```python
from build123d import *

# Parameters (mm, degrees)
CYLINDER1528_R     = 1.5
CYLINDER1528_DEPTH = 100
CYLINDER1527_R     = 1.5
CYLINDER1527_DEPTH = 100
CYLINDER1526_R     = 1.5
CYLINDER1526_DEPTH = 32
CYLINDER1525_R     = 1.5
CYLINDER1525_DEPTH = 32
BOX520_W           = 200
BOX520_H           = 100
BOX520_DEPTH       = 100
BOX519_W           = 200
BOX519_H           = 100
BOX519_DEPTH       = 100
CYLINDER1518_R     = 4
CYLINDER1518_DEPTH = 100
CYLINDER1519_R     = 4
CYLINDER1519_DEPTH = 100
CYLINDER1520_R     = 4
CYLINDER1520_DEPTH = 100
CYLINDER1521_R     = 4
CYLINDER1521_DEPTH = 100
CYLINDER1522_R     = 4
CYLINDER1522_DEPTH = 100
CYLINDER1523_R     = 4
CYLINDER1523_DEPTH = 100
CYLINDER1524_R     = 4
CYLINDER1524_DEPTH = 100
CYLINDER1517_R     = 4
CYLINDER1517_DEPTH = 100
CYLINDER1510_R     = 1.5
CYLINDER1510_DEPTH = 100
CYLINDER1511_R     = 1.5
CYLINDER1511_DEPTH = 100
CYLINDER1512_R     = 1.5
CYLINDER1512_DEPTH = 100
CYLINDER1513_R     = 1.5
CYLINDER1513_DEPTH = 100
CYLINDER1514_R     = 1.5
CYLINDER1514_DEPTH = 100
CYLINDER1515_R     = 1.5
CYLINDER1515_DEPTH = 100
CYLINDER1516_R     = 1.5
CYLINDER1516_DEPTH = 100
CYLINDER1509_R     = 1.5
CYLINDER1509_DEPTH = 100
CYLINDER1508_R     = 59
CYLINDER1508_DEPTH = 4


with BuildPart() as obj1:
    # Cylinder1528 → Cylinder1528 (new body)
    with BuildSketch(Plane(origin=(14, 0, -60), x_dir=(1, 0, 0), z_dir=(0, 0, 1))):
        Circle(CYLINDER1528_R)
    extrude(amount=CYLINDER1528_DEPTH)


with BuildPart() as obj2:
    # Cylinder1527 → Cylinder1527 (new body)
    with BuildSketch(Plane(origin=(90, 0, -60), x_dir=(1, 0, 0), z_dir=(0, 0, 1))):
        Circle(CYLINDER1527_R)
    extrude(amount=CYLINDER1527_DEPTH)

    # Compound900: union obj1
    add(obj1.part)


with BuildPart() as obj3:
    # Cylinder1526 → Cylinder1526 (new body)
    with BuildSketch(Plane(origin=(78, 41, -42), x_dir=(1, 0, 0), z_dir=(0, 0, 1))):
        Circle(CYLINDER1526_R)
    extrude(amount=CYLINDER1526_DEPTH)


with BuildPart() as compound899:
    # Cylinder1525 → Cylinder1525 (new body)
    with BuildSketch(Plane(origin=(26, 41, -42), x_dir=(1, 0, 0), z_dir=(0, 0, 1))):
        Circle(CYLINDER1525_R)
    extrude(amount=CYLINDER1525_DEPTH)

    # Compound899: union obj3
    add(obj3.part)


with BuildPart() as krychle520:
    # Box520 → Box520 (new body)
    with BuildSketch(Plane(origin=(-60, 44, -90), x_dir=(1, 0, 0), z_dir=(0, 0, 1))):
        with Locations((100, 50)):
            Rectangle(BOX520_W, BOX520_H)
    extrude(amount=BOX520_DEPTH)


with BuildPart() as krychle519:
    # Box519 → Box519 (new body)
    with BuildSketch(Plane(origin=(-60, -130, -90), x_dir=(1, 0, 0), z_dir=(0, 0, 1))):
        with Locations((100, 50)):
            Rectangle(BOX519_W, BOX519_H)
    extrude(amount=BOX519_DEPTH)


with BuildPart() as obj4:
    # Cylinder1518 → Cylinder1518 (new body)
    with BuildSketch(Plane(origin=(-16, 34, -90), x_dir=(1, 0, 0), z_dir=(0, 0, 1))):
        Circle(CYLINDER1518_R)
    extrude(amount=CYLINDER1518_DEPTH)


with BuildPart() as obj5:
    # Cylinder1519 → Cylinder1519 (new body)
    with BuildSketch(Plane(origin=(-16, -34, -90), x_dir=(1, 0, 0), z_dir=(0, 0, 1))):
        Circle(CYLINDER1519_R)
    extrude(amount=CYLINDER1519_DEPTH)


with BuildPart() as obj6:
    # Cylinder1520 → Cylinder1520 (new body)
    with BuildSketch(Plane(origin=(34, -16, -90), x_dir=(1, 0, 0), z_dir=(0, 0, 1))):
        Circle(CYLINDER1520_R)
    extrude(amount=CYLINDER1520_DEPTH)


with BuildPart() as obj7:
    # Cylinder1521 → Cylinder1521 (new body)
    with BuildSketch(Plane(origin=(16, 34, -90), x_dir=(1, 0, 0), z_dir=(0, 0, 1))):
        Circle(CYLINDER1521_R)
    extrude(amount=CYLINDER1521_DEPTH)


with BuildPart() as obj8:
    # Cylinder1522 → Cylinder1522 (new body)
    with BuildSketch(Plane(origin=(16, -34, -90), x_dir=(1, 0, 0), z_dir=(0, 0, 1))):
        Circle(CYLINDER1522_R)
    extrude(amount=CYLINDER1522_DEPTH)


with BuildPart() as obj9:
    # Cylinder1523 → Cylinder1523 (new body)
    with BuildSketch(Plane(origin=(-34, 16, -90), x_dir=(1, 0, 0), z_dir=(0, 0, 1))):
        Circle(CYLINDER1523_R)
    extrude(amount=CYLINDER1523_DEPTH)


with BuildPart() as obj10:
    # Cylinder1524 → Cylinder1524 (new body)
    with BuildSketch(Plane(origin=(34, 16, -90), x_dir=(1, 0, 0), z_dir=(0, 0, 1))):
        Circle(CYLINDER1524_R)
    extrude(amount=CYLINDER1524_DEPTH)


with BuildPart() as obj11:
    # Cylinder1517 → Cylinder1517 (new body)
    with BuildSketch(Plane(origin=(-34, -16, -90), x_dir=(1, 0, 0), z_dir=(0, 0, 1))):
        Circle(CYLINDER1517_R)
    extrude(amount=CYLINDER1517_DEPTH)

    # Compound898: union obj4, obj5, obj6, obj7, obj8, obj9, obj10
    add(obj4.part)
    add(obj5.part)
    add(obj6.part)
    add(obj7.part)
    add(obj8.part)
    add(obj9.part)
    add(obj10.part)


with BuildPart() as obj12:
    # Cylinder1510 → Cylinder1510 (new body)
    with BuildSketch(Plane(origin=(103, 12, -60), x_dir=(1, 0, 0), z_dir=(0, 0, 1))):
        Circle(CYLINDER1510_R)
    extrude(amount=CYLINDER1510_DEPTH)


with BuildPart() as obj13:
    # Cylinder1511 → Cylinder1511 (new body)
    with BuildSketch(Plane(origin=(76, 24, -60), x_dir=(1, 0, 0), z_dir=(0, 0, 1))):
        Circle(CYLINDER1511_R)
    extrude(amount=CYLINDER1511_DEPTH)


with BuildPart() as obj14:
    # Cylinder1512 → Cylinder1512 (new body)
    with BuildSketch(Plane(origin=(91, -27, -60), x_dir=(1, 0, 0), z_dir=(0, 0, 1))):
        Circle(CYLINDER1512_R)
    extrude(amount=CYLINDER1512_DEPTH)


with BuildPart() as obj15:
    # Cylinder1513 → Cylinder1513 (new body)
    with BuildSketch(Plane(origin=(13, -27, -60), x_dir=(1, 0, 0), z_dir=(0, 0, 1))):
        Circle(CYLINDER1513_R)
    extrude(amount=CYLINDER1513_DEPTH)


with BuildPart() as obj16:
    # Cylinder1514 → Cylinder1514 (new body)
    with BuildSketch(Plane(origin=(28, 24, -60), x_dir=(1, 0, 0), z_dir=(0, 0, 1))):
        Circle(CYLINDER1514_R)
    extrude(amount=CYLINDER1514_DEPTH)


with BuildPart() as obj17:
    # Cylinder1515 → Cylinder1515 (new body)
    with BuildSketch(Plane(origin=(1, -12, -60), x_dir=(1, 0, 0), z_dir=(0, 0, 1))):
        Circle(CYLINDER1515_R)
    extrude(amount=CYLINDER1515_DEPTH)


with BuildPart() as obj18:
    # Cylinder1516 → Cylinder1516 (new body)
    with BuildSketch(Plane(origin=(1, 12, -60), x_dir=(1, 0, 0), z_dir=(0, 0, 1))):
        Circle(CYLINDER1516_R)
    extrude(amount=CYLINDER1516_DEPTH)


with BuildPart() as obj19:
    # Cylinder1509 → Cylinder1509 (new body)
    with BuildSketch(Plane(origin=(103, -12, -60), x_dir=(1, 0, 0), z_dir=(0, 0, 1))):
        Circle(CYLINDER1509_R)
    extrude(amount=CYLINDER1509_DEPTH)

    # Compound897: union obj12, obj13, obj14, obj15, obj16, obj17, obj18
    add(obj12.part)
    add(obj13.part)
    add(obj14.part)
    add(obj15.part)
    add(obj16.part)
    add(obj17.part)
    add(obj18.part)


with BuildPart() as cut510:
    # Cylinder1508 → Cylinder1508 (new body)
    with BuildSketch(Plane(origin=(52, 0, -26), x_dir=(1, 0, 0), z_dir=(0, 0, 1))):
        Circle(CYLINDER1508_R)
    extrude(amount=CYLINDER1508_DEPTH)

    # Cut505: cut obj19
    add(obj19.part, mode=Mode.SUBTRACT)

    # Cut506: cut obj11
    add(obj11.part, mode=Mode.SUBTRACT)

    # Cut507: cut Krychle519
    add(krychle519.part, mode=Mode.SUBTRACT)

    # Cut508: cut Krychle520
    add(krychle520.part, mode=Mode.SUBTRACT)

    # Cut509: cut Compound899
    add(compound899.part, mode=Mode.SUBTRACT)

    # Cut510: cut obj2
    add(obj2.part, mode=Mode.SUBTRACT)


solid = cut510.part
```
Design review of the part built by this model. Coordinates are the model's own, in mm. Give positions to 0.01 mm unless a question says otherwise; leave off trailing zeros. Order: outer loops, then holes, each group sorted by start corner. A loop starts at its lowest first (then second) coordinate and runs counter-clockwise, first axis right, second up. Notation, with made-up numbers: (-19.5, 61) - (11.5, 61) arc R29 cw to (11.5, 99) - close; hole circle Ø6 at (65.25, -36.5). An arc over 180 degrees is marked (long way). Use a Markdown table: item, result. Add a question column.
(1) Add section C-C on y = -16. Give the boundary of the cut face in (x, z), then the cut area to 3 significant figures.
(2) Add section D-D on y = -27. Give the boundary of the cut face in (x, z), then the cut area to 3 significant figures.
(3) Add section B-B on z = -24.7. Give the number of separate pieces and of enclosed holes in the cut face, then the cut area to 3 significant figures.
(4) Mouldability with a two-part tool opening along Y and no side actions: class faces 1 (the face through (51, 8, -26)), 2 (the face through (110.385, 8.496, -24.028)), 3 (the face through (15.479, 37.966, -24.028)) as +Y half, -Y half, draft (parallel to the pull), parting line (faces both ways), or undercut.
(5) Wall thickness on probe 1 along X at (y, z) = (0, -23.3); probe 2 along Y at (x, z) = (34, -24.15); probe 3 along Y at (x, z) = (1, -24.1): over which ranges is each line inside the solid? List them lowest first. Write a range as [from, to].
(6) Clearance check with a flat-ended pin moving along its axis: P1, Ø1.8, axis at x = 103, y = 12, coming from the +Z side. State where the tip first meets the part, or that it passes through.
(7) Add section A-A on x = 34. Give the boundary of the cut face in (y, z).
Report:
| question | item | result |
|---|---|---|
| 1 | outline | (-4.79, -26) - (30, -26) - (30, -22) - (-4.79, -22) - close; (38, -26) - (108.79, -26) - (108.79, -22) - (38, -22) - close |
| 1 | area | 422 mm² |
| 2 | outline | (-0.46, -26) - (11.5, -26) - (11.5, -22) - (-0.46, -22) - close; (14.5, -26) - (89.5, -26) - (89.5, -22) - (14.5, -22) - close; (92.5, -26) - (104.46, -26) - (104.46, -22) - (92.5, -22) - close |
| 2 | area | 396 mm² |
| 3 | separate pieces | 1 |
| 3 | enclosed holes | 15 |
| 3 | area | 7,800 mm² |
| 4 | face 1 | draft |
| 4 | face 2 | parting line |
| 4 | face 3 | undercut |
| 5 | probe 1 | x = [-7, 12.5], [15.5, 88.5], [91.5, 111] |
| 5 | probe 2 | y = [-30, -20], [-12, 12], [20, 44] |
| 5 | probe 3 | y = [-29.66, -13.5], [-10.5, 10.5], [13.5, 29.66] |
| 6 | P1 | passes through |
| 7 | outline | (-30, -26) - (-20, -26) - (-20, -22) - (-30, -22) - close; (-12, -26) - (12, -26) - (12, -22) - (-12, -22) - close; (20, -26) - (44, -26) - (44, -22) - (20, -22) - close |
